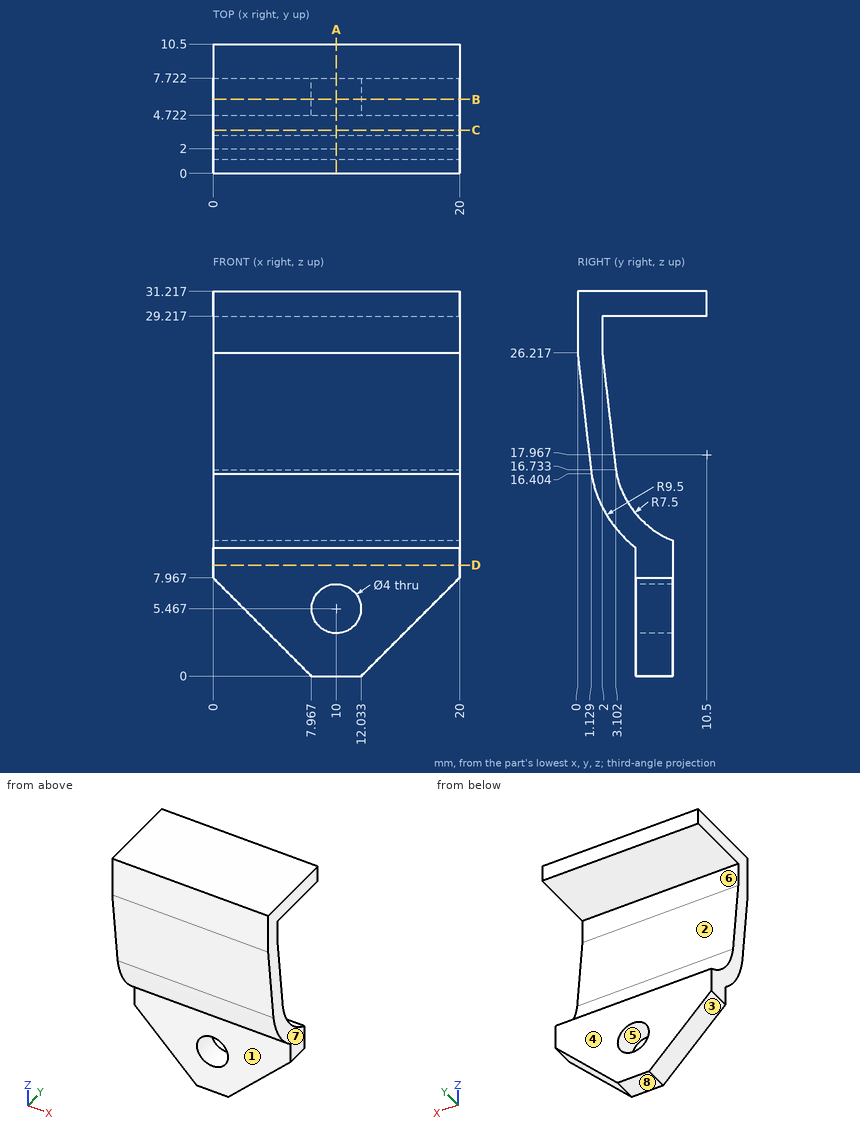
For this review, use the dimensioned drawing (mm, ordinates from the lowest corner) and the shaded views. A direction names the side the tool comes from. Round coordinates to 2 decimals unless told otherwise and drop trailing zeros. Write each loop counter-clockwise with the first axis right and the second up, starting at its lowest first coordinate (ties: lowest second). Pieces come first, ordered by that corner, then holes. Notation, with made-up numbers: M 3.5,75 L 27.5,75 A32 ccw 27.5,108 Z; hole C -39,48 d6. An arc over 180 degrees is marked long. Answer as CSV lines item,"result". Start each with the question number.
Q1. Consider section C-C, the plane y = 3.5. Give the boundary of the cut face in (x, z).
Q2. The part is to be moulded in two halves that separate along Z. For the marked faces 6, 7 and 8, say which applies: +Z half, -Z half, draft (parallel to the pull), parting line (faces both ways), or undercut.
Q3. Consider section D-D, the plane z = 9. Give the boundary of the cut face in (x, y).
Q4. Clearance check with flat-ended pins moving along their axes: P1, Ø6.5, axis at x = 10, z = 5.47, coming from the +Y side; P2, Ø4, axis at y = 5.5, z = 4.5, coming from the -X side (1 decimal); P3, Ø11.5, axis at x = 14.5, z = 3.5, coming from the -Y side. State where each tip first meets the part, or that it passes through.
Q5. Wall thickness on line 1 along Z through (x, y) = (10, 6.75) (1 decimal); line 2 along Z through (x, y) = (10, 5.85) (1 decimal); line 3 along Y through (x, z) = (11.5, 29): over which ranges is each line inside the solid? List them lowest first.
Q6. Tool access review of the marked faces 1, 2, 3, 4 and 5: name each direction out of +Z, -Z, +X, -X, +Y, -Y from which nothing blocks a thin tool from reaching the whole face with its end or side.
Q7. Consider section B-B, the plane y = 6. Give the boundary of the cut face in (x, z).
Q8. Consider section A-A, the plane x = 10. Give the boundary of the cut face in (y, z) (1 decimal).
Result set:
1,outline,"M 0,11.54 L 20,11.54 L 20,15.27 L 0,15.27 Z; M 0,29.22 L 20,29.22 L 20,31.22 L 0,31.22 Z"
2,face 6,"undercut"
2,face 7,"draft"
2,face 8,"-Z half"
3,outline,"M 0,4.72 L 20,4.72 L 20,7.72 L 0,7.72 Z"
4,P1,"stops at y = 7.72"
4,P2,"stops at x = 1.5"
4,P3,"stops at y = 4.72"
5,line 1,"z = 0 to 3.5, 7.5 to 11.5, 29.2 to 31.2"
5,line 2,"z = 0 to 3.5, 7.5 to 12.1, 29.2 to 31.2"
5,line 3,"y = 0 to 2"
6,face 1,"-Z, +X, -X, -Y"
6,face 2,"+X, -X, +Y"
6,face 3,"-Z, -X, +Y, -Y"
6,face 4,"-Z, +X, -X, +Y"
6,face 5,"+Y, -Y"
7,outline,"M 0,7.97 L 7.97,0 L 12.03,0 L 20,7.97 L 20,11.97 L 0,11.97 Z; M 0,29.22 L 20,29.22 L 20,31.22 L 0,31.22 Z; hole C 10,5.47 d4"
8,outline,"M 0,26.2 L 1.1,16.4 A9.5 ccw 4.7,10.4 L 4.7,7.5 L 7.7,7.5 L 7.7,11 A7.5 cw 3.1,16.7 L 2,26.2 L 2,29.2 L 10.5,29.2 L 10.5,31.2 L 0,31.2 Z; M 4.7,0 L 7.7,0 L 7.7,3.5 L 4.7,3.5 Z"
